Input: part model. Units: mm. Frame: model coordinates. Coordinates: 2 decimals unless noted, no trailing zeros. Loops run counter-clockwise (first coordinate to the right, second up) from the corner with the lowest first, then second, coordinate; pieces in that order, holes last. Notation, with made-up numbers: (25, 84) - (77, 84) arc R12 cw to (77, 105) - close; hole circle Ø9 at (11.25, 41.5). An arc over 180 degrees is marked (long way). Answer as CSV lines item,"result". Start each with the question number.
```python
from build123d import *

# Parameters (mm, degrees)
F1_DEPTH       = 2020
F3_D           = 6
F3_CBORE_D     = 9.5
F3_CBORE_DEPTH = 8.5


with BuildPart() as f1:
    # F0 (on Right) → F1 (new body)
    with BuildSketch(Plane.YZ):
        with BuildLine():
            Line((-3, 0.5), (0, 0.5))
            Line((0, 0.5), (3, 0.5))
            Line((3, 0.5), (3.5, 0))
            Line((3.5, 0), (9.5, 0))
            Line((9.5, 0), (10, 0.5))
            Line((10, 0.5), (10, 4.6))
            Line((10, 4.6), (7.525126, 7.074874))
            Line((7.525126, 7.074874), (7.525126, 9.550253))
            Line((7.525126, 9.550253), (7.701903, 9.727029))
            ThreePointArc((7.701903, 9.727029), (8.40901, 11.141243), (9.823223, 11.84835))
            Line((9.823223, 11.84835), (10, 12.025126))
            Line((10, 12.025126), (10, 14.025126))
            Line((10, 14.025126), (9.823223, 14.201903))
            ThreePointArc((9.823223, 14.201903), (8.40901, 14.90901), (7.701903, 16.323223))
            Line((7.701903, 16.323223), (7.525126, 16.5))
            Line((7.525126, 16.5), (0, 16.5))
            Line((0, 16.5), (-7.525126, 16.5))
            Line((-7.525126, 16.5), (-7.701903, 16.323223))
            ThreePointArc((-7.701903, 16.323223), (-8.40901, 14.90901), (-9.823223, 14.201903))
            Line((-9.823223, 14.201903), (-10, 14.025126))
            Line((-10, 14.025126), (-10, 12.025126))
            Line((-10, 12.025126), (-9.823223, 11.84835))
            ThreePointArc((-9.823223, 11.84835), (-8.40901, 11.141243), (-7.701903, 9.727029))
            Line((-7.701903, 9.727029), (-7.525126, 9.550253))
            Line((-7.525126, 9.550253), (-7.525126, 7.074874))
            Line((-7.525126, 7.074874), (-10, 4.6))
            Line((-10, 4.6), (-10, 0.5))
            Line((-10, 0.5), (-9.5, 0))
            Line((-9.5, 0), (-3.5, 0))
            Line((-3.5, 0), (-3, 0.5))
        make_face()
    extrude(amount=F1_DEPTH)

    # F3 (through all)
    with Locations(Plane.XY.offset(16.5)):
        with Locations((20, 0), (80, 0), (140, 0), (200, 0), (260, 0), (320, 0), (380, 0), (500, 0), (440, 0), (560, 0), (620, 0), (680, 0), (740, 0), (800, 0), (860, 0), (920, 0), (980, 0), (1040, 0), (1100, 0), (1160, 0), (1220, 0), (1280, 0), (1340, 0), (1400, 0), (1460, 0), (1520, 0), (1580, 0), (1640, 0), (1700, 0), (1760, 0), (1820, 0), (1880, 0), (1940, 0), (2000, 0)):
            CounterBoreHole(F3_D / 2, F3_CBORE_D / 2, F3_CBORE_DEPTH)


solid = f1.part
```
Item 1: Material intervals for probe 1 along Y at (x, z) = (1100, 3.5); probe 2 along Y at (x, z) = (1340, 10.5); probe 3 along Z at (x, y) = (996.5, -1), sorted ascending.
Item 2: Contact query for a flat-ended pin moving along its axis: P1, Ø1.8, axis at x = 712.5, y = 1, coming from the -Z side. Output: stop coordinate, or through.
Item 3: Section query A-A, the plane x = 1250.5. Output: boundary loops of the cut face in (y, z).
Response values:
1,probe 1,"y = -10 to -3, 3 to 10"
1,probe 2,"y = -7.94 to -4.75, 4.75 to 7.94"
1,probe 3,"z = 0.5 to 16.5"
2,P1,"stops at z = 0.5"
3,outline,"(-10, 0.5) - (-9.5, 0) - (-3.5, 0) - (-3, 0.5) - (3, 0.5) - (3.5, 0) - (9.5, 0) - (10, 0.5) - (10, 4.6) - (7.53, 7.07) - (7.53, 9.55) - (7.7, 9.73) arc R2.5 cw to (9.82, 11.85) - (10, 12.03) - (10, 14.03) - (9.82, 14.2) arc R2.5 cw to (7.7, 16.32) - (7.53, 16.5) - (-7.53, 16.5) - (-7.7, 16.32) arc R2.5 cw to (-9.82, 14.2) - (-10, 14.03) - (-10, 12.03) - (-9.82, 11.85) arc R2.5 cw to (-7.7, 9.73) - (-7.53, 9.55) - (-7.53, 7.07) - (-10, 4.6) - close"
